Here's how the part is built. I have some questions about the finished solid (model axes, mm). Coordinates: 2 decimals unless noted, no trailing zeros. Write each loop counter-clockwise with the first axis right and the second up, starting at its lowest first coordinate (ties: lowest second). Pieces come first, ordered by that corner, then holes.
(1) For pin 1 Ø3 at (x, y) = (-19, -34) entering from -Z; pin 2 Ø1 at (x, z) = (12, -9.5) entering from +Y; pin 3 Ø1 at (x, y) = (13, 26) entering from -Z; pin 4 Ø4 at (x, z) = (9, -12.5) entering from -Y, each with a flat end and sliding along its axis, tell me the tip position at first contact or that it passes through.
(2) Imagine slicing it at A-A, the plane x = 0. List the corners of the cut face in (y, z) for me.
(3) Please list where these lines run through material, in increasing order: probe 1 along Y at (x, z) = (0, 2.85); probe 2 along X at (y, z) = (-10.5, 3.1); probe 3 along Y at (x, z) = (0, -10).
(4) Imagine slicing it at C-C, the plane y = 13.5. List the corners of the cut face in (x, z) for me.
(5) Thinking about a two-plate mould opening in Y: for faces 1 (the cylindrical face through (-18.798, 32.463, 2.535)), 2 (the flat face through (0, 9, 0)), 3 (the cylindrical face through (3.64, -26.9, -9.3)), which applies, released by +Y, released by -Y, zero draft, split by the parting line, or undercut?
(6) Imagine slicing it at B-B, the plane z = -12.5. List the corners of the cut face in (x, y) for me.
```python
from build123d import *

# Parameters (mm, degrees)
SKETCH1_W           = 45
SKETCH1_H           = 75
BOSS_EXTRUDE1_DEPTH = 5
SKETCH2_R           = 1.55
SKETCH2_R_2         = 14.5
SKETCH2_R_3         = 10
CUT_EXTRUDE4_DEPTH  = 27.5
FILLET3_R           = 4
SKETCH3_R           = 16.8
SKETCH3_R_2         = 14.5
BOSS_EXTRUDE2_DEPTH = 16.8
FILLET4_R           = 2
FILLET5_R           = 1


with BuildPart() as part:
    # Sketch1 → Boss-Extrude1 (new body)
    with BuildSketch(Plane.XY):
        Rectangle(SKETCH1_W, SKETCH1_H)
    extrude(amount=BOSS_EXTRUDE1_DEPTH)

    # Sketch2 → Cut-Extrude4 (cut, symmetric)
    # profile 1 of 6: a face of its own
    with BuildSketch(Plane.XY.offset(5)):
        with Locations(Location((19, 34, 0), (0, 0, 180))):
            Circle(SKETCH2_R)
    # profile 2 of 6: a face of its own
    with BuildSketch(Plane.XY.offset(5)):
        with Locations(Location((-19, 34, 0), (0, 0, 180))):
            Circle(SKETCH2_R)
    # profile 3 of 6: a face of its own
    with BuildSketch(Plane.XY.offset(5)):
        with Locations(Location((19, -34, 0), (0, 0, 180))):
            Circle(SKETCH2_R)
    # profile 4 of 6: a face of its own
    with BuildSketch(Plane.XY.offset(5)):
        with Locations(Location((-19, -34, 0), (0, 0, 180))):
            Circle(SKETCH2_R)
    # profile 5 of 6: a face of its own
    with BuildSketch(Plane.XY.offset(5)):
        with Locations(Location((0, -10.5, 0), (0, 0, 180))):
            Circle(SKETCH2_R_2)
        with Locations((0, -10.5)):
            Circle(SKETCH2_R_3, mode=Mode.SUBTRACT)
    # profile 6 of 6: a face of its own
    with BuildSketch(Plane.XY.offset(5)):
        with Locations((0, -10.5)):
            Circle(SKETCH2_R_3)
    extrude(amount=CUT_EXTRUDE4_DEPTH, both=True, mode=Mode.SUBTRACT)

    # Fillet3
    fillet3_edges = [part.edges().sort_by_distance(p)[0] for p in [
        (-22.5, -37.5, 2.5),
        (-22.5, 37.5, 2.5),
        (22.5, 37.5, 2.5),
        (22.5, -37.5, 2.5),
    ]]
    fillet(fillet3_edges, radius=FILLET3_R)

    # Sketch3 → Boss-Extrude2 (add)
    with BuildSketch(Plane(origin=(0, 0, 0), x_dir=(-1, 0, 0), z_dir=(0, 0, -1))):
        with Locations((0, -10.5)):
            Circle(SKETCH3_R)
        with Locations((0, -10.5)):
            Circle(SKETCH3_R_2, mode=Mode.SUBTRACT)
    extrude(amount=BOSS_EXTRUDE2_DEPTH)

    # Fillet4
    fillet4_edges = [part.edges().sort_by_distance(p)[0] for p in [
        (16.8, -10.5, 0),
    ]]
    fillet(fillet4_edges, radius=FILLET4_R)

    # Fillet5
    fillet5_edges = [part.edges().sort_by_distance(p)[0] for p in [
        (14.5, -10.5, 5),
        (0, -37.5, 0),
        (-22.5, 0, 0),
        (0, 37.5, 0),
        (22.5, 0, 0),
        (-21.328427125, 36.328427125, 0),
        (21.328427125, 36.328427125, 0),
        (21.328427125, -36.328427125, 0),
        (-21.328427125, -36.328427125, 0),
    ]]
    fillet(fillet5_edges, radius=FILLET5_R)


solid = part.part
```
Recorded:
1. pin 1: passes through
1. pin 2: stops at y = 1.75
1. pin 3: stops at z = 0
1. pin 4: stops at y = -25.77
2. outline: (-37.5, 1) arc R1 ccw to (-36.5, 0) - (-29.3, 0) arc R2 cw to (-27.3, -2) - (-27.3, -16.8) - (-25, -16.8) - (-25, 4) arc R1 ccw to (-26, 5) - (-37.5, 5) - close; (4, -16.8) - (6.3, -16.8) - (6.3, -2) arc R2 cw to (8.3, 0) - (36.5, 0) arc R1 ccw to (37.5, 1) - (37.5, 5) - (5, 5) arc R1 ccw to (4, 4) - close
3. probe 1: y = -37.5 to -25, 4 to 37.5
3. probe 2: x = -22.5 to -14.5, 14.5 to 22.5
3. probe 3: y = -27.3 to -25, 4 to 6.3
4. outline: (-22.5, 1) arc R1 ccw to (-21.5, 0) - (21.5, 0) arc R1 ccw to (22.5, 1) - (22.5, 5) - (-22.5, 5) - close
5. face 1: undercut
5. face 2: zero draft
5. face 3: split by the parting line
6. outline: circle Ø33.6 at (0, -10.5); hole circle Ø29 at (0, -10.5)
